Model file for the job. Use its own axes, mm. A direction names the side the tool comes from. Coordinates: 2 decimals unless noted, no trailing zeros. Loops run counter-clockwise (first coordinate to the right, second up) from the corner with the lowest first, then second, coordinate; pieces in that order, holes last.
from build123d import *

# Parameters (mm, degrees)
SKIZZE1_W                            = 640
SKIZZE1_H                            = 430
AUFSATZ_LINEAR_AUSTRAGEN1_DEPTH      = 185
VERRUNDUNG1_R                        = 150
SCHNITT_LINEAR_AUSTRAGEN1_DEPTH      = 186
SCHNITT_LINEAR_AUSTRAGEN1_DRAFT      = 2
SCHNITT_LINEAR_AUSTRAGEN_D_NN1_DEPTH = 10


with BuildPart() as part:
    # Skizze1 → Aufsatz-Linear austragen1 (new body)
    with BuildSketch(Plane(origin=(0, 0, 0), x_dir=(1, 0, 0), z_dir=(0, 1, 0))):
        with Locations((320, 215)):
            Rectangle(SKIZZE1_W, SKIZZE1_H)
    extrude(amount=AUFSATZ_LINEAR_AUSTRAGEN1_DEPTH)

    # Verrundung1
    verrundung1_edges = [part.edges().sort_by_distance(p)[0] for p in [
        (0, 92.5, -430),
        (640, 92.5, -430),
    ]]
    fillet(verrundung1_edges, radius=VERRUNDUNG1_R)


with BuildPart() as schnitt_linear_austragen1_tool:
    # Skizze2 → Schnitt-Linear austragen1 (with draft: the straight prism first)
    with BuildSketch(Plane(origin=(0, 185, 0), x_dir=(1, 0, 0), z_dir=(0, 1, 0))):
        with BuildLine():
            Line((490, 400), (435, 400))
            Line((435, 400), (435, 405))
            Line((435, 405), (205, 405))
            Line((205, 405), (205, 400))
            Line((205, 400), (150, 400))
            ThreePointArc((150, 400), (65.147186258, 364.852813742), (30, 280))
            Line((30, 280), (30, 30))
            Line((30, 30), (205, 30))
            Line((205, 30), (205, 25))
            Line((205, 25), (435, 25))
            Line((435, 25), (435, 30))
            Line((435, 30), (610, 30))
            Line((610, 30), (610, 280))
            ThreePointArc((610, 280), (574.852813742, 364.852813742), (490, 400))
        make_face()
    extrude(amount=-SCHNITT_LINEAR_AUSTRAGEN1_DEPTH)
    # Schnitt-Linear austragen1: the draft: its side faces are tilted about the plane it starts from
    schnitt_linear_austragen1_sides = [schnitt_linear_austragen1_tool.faces().sort_by_distance(p)[0] for p in [
        (462.5, 92, -400),
        (435, 92, -402.5),
        (320, 92, -405),
        (205, 92, -402.5),
        (177.5, 92, -400),
        (65.147186258, 92, -364.852813742),
        (30, 92, -155),
        (117.5, 92, -30),
        (205, 92, -27.5),
        (320, 92, -25),
        (435, 92, -27.5),
        (522.5, 92, -30),
        (610, 92, -155),
        (574.852813742, 92, -364.852813742),
    ]]
    draft(schnitt_linear_austragen1_sides, Plane(origin=(0, 185, 0), x_dir=(1, 0, 0), z_dir=(0, 1, 0)), SCHNITT_LINEAR_AUSTRAGEN1_DRAFT)


with BuildPart() as part_1:
    add(part.part)

    # Schnitt-Linear austragen1: cut by schnitt_linear_austragen1_tool
    add(schnitt_linear_austragen1_tool.part, mode=Mode.SUBTRACT)

    # Skizze3 → Schnitt-Linear-Austragen-Dünn1 (cut)
    with BuildSketch(Plane(origin=(0, 185, 0), x_dir=(1, 0, 0), z_dir=(0, 1, 0))):
        with BuildLine():
            Line((490, 422), (150, 422))
            ThreePointArc((150, 422), (49.590837072, 380.409162928), (8, 280))
            Line((8, 280), (8, 8))
            Line((8, 8), (632, 8))
            Line((632, 8), (632, 280))
            ThreePointArc((632, 280), (590.409162928, 380.409162928), (490, 422))
        make_face()
        with BuildLine():
            Line((490, 412), (150, 412))
            ThreePointArc((150, 412), (56.661904883, 373.338095117), (18, 280))
            Line((18, 280), (18, 18))
            Line((18, 18), (622, 18))
            Line((622, 18), (622, 280))
            ThreePointArc((622, 280), (583.338095117, 373.338095117), (490, 412))
        make_face(mode=Mode.SUBTRACT)
    extrude(amount=-SCHNITT_LINEAR_AUSTRAGEN_D_NN1_DEPTH, mode=Mode.SUBTRACT)


solid = part_1.part
Q1. Flat gauge pins, fed straight in: P1, Ø1.5, axis at x = 65.5, y = 89.5, coming from the -Z side; P2, Ø8, axis at x = 573, y = 152.5, coming from the -Z side. Where does each tip first touch, or does it go through?
Answers:
P1: stops at z = -404.44
P2: stops at z = -407.51
Q2. Mould opens along Z. For faces 1 (the flat face through (0, 91, -138)), 2 (the conical face through (578.1, 93.8, -366.1)), 3 (the flat face through (318, 91, -430)) say: +Z half, -Z half, draft (parallel to the pull), parting line (faces both ways), or undercut.
Answers:
face 1: draft
face 2: undercut
face 3: -Z half
Q3. Slice it at A-A (x = 223). List the corners of the cut face in (y, z), and give its area (3 significant figures).
Answers:
outline: (0, -430) - (185, -430) - (185, -422) - (175, -422) - (175, -412) - (185, -412) - (185, -405) - (0, -411.46) - close; (0, -18.54) - (185, -25) - (185, -18) - (175, -18) - (175, -8) - (185, -8) - (185, 0) - (0, 0) - close
area: 7,850 mm2
Q4. Drill centre lines: line 1 (X direction, y = 176, z = -336.5); line 2 (Z direction, x = 396.5, y = 27); line 3 (X direction, y = 107, z = -23.5). Where is each one in solid material? Low to high.
Answers:
line 1: x = 11.05 to 19.72, 30.7 to 43.78, 596.22 to 609.3, 620.28 to 628.95
line 2: z = -430 to -410.52, -19.48 to 0
line 3: x = 0 to 202.28, 437.72 to 640
Q5. Slice it at B-B (z = -233). List the corners of the cut face in (x, y), and give its area (3 significant figures).
Answers:
outline: (0, 0) - (23.54, 0) - (30, 185) - (18, 185) - (18, 175) - (8, 175) - (8, 185) - (0, 185) - close; (610, 185) - (616.46, 0) - (640, 0) - (640, 185) - (632, 185) - (632, 175) - (622, 175) - (622, 185) - close
area: 9,700 mm2
Q6. Which spindle directions (+Z, -Z, +X, -X, +Y, -Y) get a long thin tool onto all of the face, cutting with end or side? Do faces 4 (the conical face through (63.9, 93.8, -368.1)), 5 (the cylindrical face through (57.694, 180.07, -374.359)), 6 (the flat face through (319, 185, -423)). Say none if no direction does.
Answers:
face 4: -Y
face 5: +Y
face 6: +Z, -Z, +X, -X, +Y
Q7. Slice it at C-C (y = 78.5). List the corners of the cut face in (x, z).
Answers:
outline: (0, -280) arc R150 ccw to (150, -430) - (490, -430) arc R150 ccw to (640, -280) - (640, 0) - (0, 0) - close; hole (26.28, -280) arc R123.72 ccw to (150, -403.72) - (201.28, -403.72) - (201.28, -408.72) - (438.72, -408.72) - (438.72, -403.72) - (490, -403.72) arc R123.72 ccw to (613.72, -280) - (613.72, -26.28) - (438.72, -26.28) - (438.72, -21.28) - (201.28, -21.28) - (201.28, -26.28) - (26.28, -26.28) - close
Q8. Slice it at D-D (y = 145). List the corners of the cut face in (x, z).
Answers:
outline: (0, -280) arc R150 ccw to (150, -430) - (490, -430) arc R150 ccw to (640, -280) - (640, 0) - (0, 0) - close; hole (28.6, -280) arc R121.4 ccw to (150, -401.4) - (203.6, -401.4) - (203.6, -406.4) - (436.4, -406.4) - (436.4, -401.4) - (490, -401.4) arc R121.4 ccw to (611.4, -280) - (611.4, -28.6) - (436.4, -28.6) - (436.4, -23.6) - (203.6, -23.6) - (203.6, -28.6) - (28.6, -28.6) - close
